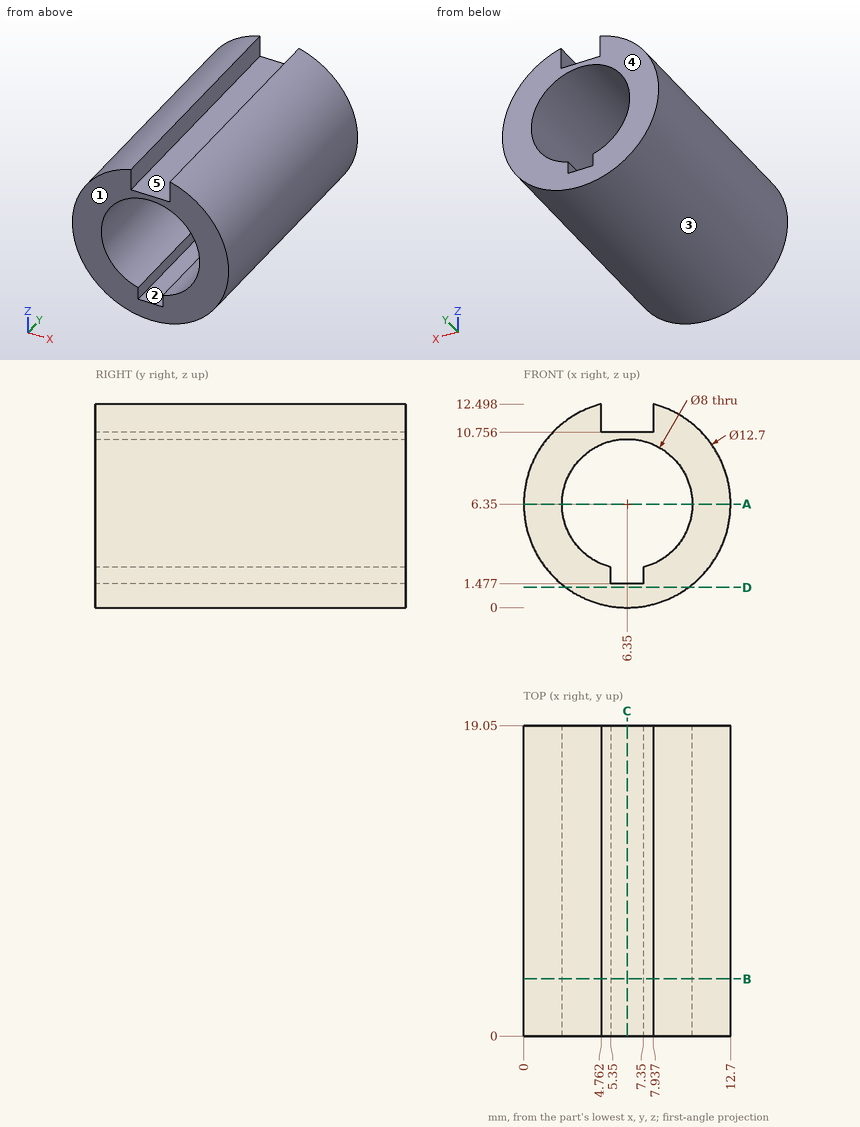
Print and shaded views of the part. All mm, measured from the part's lowest x, y and z. A direction names the side the tool comes from. Give positions to 0.01 mm unless a question says otherwise; leave off trailing zeros. Write each loop counter-clockwise with the first axis right and the second up, starting at its lowest first coordinate (ties: lowest second). Pieces come first, ordered by that corner, then holes. Notation, with made-up numbers: M -14.5,72 L 0.5,72 A18 ccw 0.5,94 Z; hole C -5,62.25 d2. An arc over 180 degrees is marked long. Use a Markdown table: item, result.
1) Cut at C-C (x = 6.35). List the corners of the cut face in (y, z).
Responses:
| item | result |
|---|---|
| outline | M 0,0 L 19.05,0 L 19.05,1.48 L 0,1.48 Z; M 0,10.35 L 19.05,10.35 L 19.05,10.76 L 0,10.76 Z |
2) Pull direction X, two halves, no side cores. Call the marked faces 1, 2 and 3: +X half, -X half, draft (parallel to the pull), parting line (faces both ways), or undercut.
Responses:
| item | result |
|---|---|
| face 1 | draft |
| face 2 | undercut |
| face 3 | parting line |
3) Cut at B-B (y = 3.5). List the corners of the cut face in (x, z).
Responses:
| item | result |
|---|---|
| outline | M 4.76,10.76 L 4.76,12.5 A6.35 ccw long 7.94,12.5 L 7.94,10.76 Z; hole M 5.35,1.48 L 7.35,1.48 L 7.35,2.48 A4 ccw long 5.35,2.48 Z |
4) Cut at D-D (z = 1.25). List the corners of the cut face in (x, y), and give its area (3 significant figures).
Responses:
| item | result |
|---|---|
| outline | M 2.57,0 L 10.13,0 L 10.13,19.05 L 2.57,19.05 Z |
| area | 144 mm2 |
5) Drill centre lines: line 1 (X direction, y = 11, z = 6.35); line 2 (Z direction, x = 8.5, y = 15.75) (1 decimal); line 3 (Z direction, x = 6.35, y = 13.25). Where is each one in solid material? Low to high. Write a range as from..to.
Responses:
| item | result |
|---|---|
| line 1 | x = 0..2.35, 10.35..12.7 |
| line 2 | z = 0.4..3, 9.7..12.3 |
| line 3 | z = 0..1.48, 10.35..10.76 |
6) Pin check, flat tips, straight feed: pin 1 (1.9 mm diameter, centred on y = 7.5, z = 12, fed in from +X); pin 2 (1.5 mm diameter, centred on y = 7, z = 10, fed in from +X); pin 3 (0.5 mm diameter, centred on y = 12.5, z = 11.5, fed in from -X); pin 4 (1.5 mm diameter, centred on x = 4.5, z = 6.5, fed in from +Y). Stop position of each tip, or through.
Responses:
| item | result |
|---|---|
| pin 1 | stops at x = 10.62 |
| pin 2 | stops at x = 12 |
| pin 3 | stops at x = 2.31 |
| pin 4 | passes through |
7) Cut at A-A (z = 6.35). List the corners of the cut face in (x, y).
Responses:
| item | result |
|---|---|
| outline | M 0,0 L 2.35,0 L 2.35,19.05 L 0,19.05 Z; M 10.35,0 L 12.7,0 L 12.7,19.05 L 10.35,19.05 Z |
8) Tool access for the marked faces 4 and 5: list every direction of +Z, -Z, +X, -X, +Y, -Y with a clear straight run to the whole face (end or side of a thin tool).
Responses:
| item | result |
|---|---|
| face 4 | +Z, -Z, +X, -X, +Y |
| face 5 | +Z, +Y, -Y |
